The model under review builds one solid part; all positions refer to its coordinate system, in mm. A direction names the side the tool comes from. Give positions to 0.01 mm unless a question says otherwise; leave off trailing zeros. Write each loop counter-clockwise with the first axis right and the second up, starting at its lowest first coordinate (ties: lowest second). Pieces come first, ordered by that corner, then holes. Notation, with made-up numbers: M 25.25,28.25 L 70.25,28.25 A21 ccw 70.25,37.25 Z; hole C -26,41.5 d8. An arc over 180 degrees is marked long. Write item = value, one per line. Start each with the question number.
```python
from build123d import *

# Parameters (mm, degrees)
F0_R        = 1.75
F1_DEPTH    = 1.524
F2_R        = 6.985
F3_T1_DEPTH = 26.7357127365
F4_R        = 4.7625
F5_DEPTH    = 25.4


# Not quite as in the source:
# - a fillet or chamfer that OpenCascade refuses, or shapes differently, is made with other operations: its cross-section is extruded or revolved along the edge and cut away or added


with BuildPart() as f1:
    # F0 (on Top) → F1 (new body)
    with BuildSketch(Plane.XY):
        Polygon((3.175, 3.175), (3.175, 14.2875), (-3.175, 14.2875), (-3.175, 3.175), (-14.2875, 3.175), (-14.2875, -3.175), (-3.175, -3.175), (-3.175, -14.2875), (3.175, -14.2875), (3.175, -3.175), (14.2875, -3.175), (14.2875, 3.175), align=None)
        with BuildLine():
            ThreePointArc((1.75, -9.525), (-1.2374368671, -10.7624368671), (0, -7.775))
            ThreePointArc((0, -7.775), (1.2374368671, -8.2875631329), (1.75, -9.525))
        make_face(mode=Mode.SUBTRACT)
        with Locations((-7.9375, 0)):
            Circle(F0_R, mode=Mode.SUBTRACT)
        with BuildLine():
            ThreePointArc((9.6875, 0), (7.9375, -1.75), (6.1875, 0))
            ThreePointArc((6.1875, 0), (7.9375, 1.75), (9.6875, 0))
        make_face(mode=Mode.SUBTRACT)
        with BuildLine():
            ThreePointArc((0, 7.775), (-1.2374368671, 10.7624368671), (1.75, 9.525))
            ThreePointArc((1.75, 9.525), (1.2374368671, 8.2875631329), (0, 7.775))
        make_face(mode=Mode.SUBTRACT)
    extrude(amount=F1_DEPTH)

    # F2
    f2_edges = [f1.edges().sort_by_distance(p)[0] for p in [
        (3.175, -3.175, 0.762),
        (-3.175, 3.175, 0.762),
        (3.175, 3.175, 0.762),
        (-3.175, -3.175, 0.762),
    ]]
    fillet(f2_edges, radius=F2_R)

    # F3: fillet of radius 5.08 on 8 edges, made by hand

    # F3_s2 → F3_t1 (cut)
    with BuildSketch(Plane.XY.offset(-12.6058563682)):
        with BuildLine():
            ThreePointArc((3.1968016831, 9.6085526316), (1.5800515868, 12.9387027128), (-1.8673425473, 14.2875))
            Line((-1.8673425473, 14.2875), (-1.8673425473, 14.7955))
            Line((-1.8673425473, 14.7955), (3.175, 14.7955))
            Line((3.175, 14.7955), (3.683, 14.2875))
            ThreePointArc((3.683, 14.2875), (3.683, 10.16), (3.7032161062, 9.6486578947))
            Line((3.7032161062, 9.6486578947), (3.1968016831, 9.6085526316))
        make_face()
        with BuildLine():
            ThreePointArc((1.8673425473, 14.2875), (-1.5800515868, 12.9387027128), (-3.1968016831, 9.6085526316))
            Line((-3.1968016831, 9.6085526316), (-3.7032161062, 9.6486578947))
            ThreePointArc((-3.7032161062, 9.6486578947), (-3.683, 10.16), (-3.683, 14.2875))
            Line((-3.683, 14.2875), (-3.175, 14.7955))
            Line((-3.175, 14.7955), (1.8673425473, 14.7955))
            Line((1.8673425473, 14.7955), (1.8673425473, 14.2875))
        make_face()
        with BuildLine():
            ThreePointArc((-14.2875, 1.8673425473), (-12.9387027128, -1.5800515868), (-9.6085526316, -3.1968016831))
            Line((-9.6085526316, -3.1968016831), (-9.6486578947, -3.7032161062))
            ThreePointArc((-9.6486578947, -3.7032161062), (-10.16, -3.683), (-14.2875, -3.683))
            Line((-14.2875, -3.683), (-14.7955, -3.175))
            Line((-14.7955, -3.175), (-14.7955, 1.8673425473))
            Line((-14.7955, 1.8673425473), (-14.2875, 1.8673425473))
        make_face()
        with BuildLine():
            ThreePointArc((-9.6085526316, 3.1968016831), (-12.9387027128, 1.5800515868), (-14.2875, -1.8673425473))
            Line((-14.2875, -1.8673425473), (-14.7955, -1.8673425473))
            Line((-14.7955, -1.8673425473), (-14.7955, 3.175))
            Line((-14.7955, 3.175), (-14.2875, 3.683))
            ThreePointArc((-14.2875, 3.683), (-10.16, 3.683), (-9.6486578947, 3.7032161062))
            Line((-9.6486578947, 3.7032161062), (-9.6085526316, 3.1968016831))
        make_face()
        with BuildLine():
            ThreePointArc((1.8673425473, -14.2875), (-1.5800515868, -12.9387027128), (-3.1968016831, -9.6085526316))
            Line((-3.1968016831, -9.6085526316), (-3.7032161062, -9.6486578947))
            ThreePointArc((-3.7032161062, -9.6486578947), (-3.683, -10.16), (-3.683, -14.2875))
            Line((-3.683, -14.2875), (-3.175, -14.7955))
            Line((-3.175, -14.7955), (1.8673425473, -14.7955))
            Line((1.8673425473, -14.7955), (1.8673425473, -14.2875))
        make_face()
        with BuildLine():
            ThreePointArc((3.1968016831, -9.6085526316), (1.5800515868, -12.9387027128), (-1.8673425473, -14.2875))
            Line((-1.8673425473, -14.2875), (-1.8673425473, -14.7955))
            Line((-1.8673425473, -14.7955), (3.175, -14.7955))
            Line((3.175, -14.7955), (3.683, -14.2875))
            ThreePointArc((3.683, -14.2875), (3.683, -10.16), (3.7032161062, -9.6486578947))
            Line((3.7032161062, -9.6486578947), (3.1968016831, -9.6085526316))
        make_face()
        with BuildLine():
            ThreePointArc((14.2875, 1.8673425473), (12.9387027128, -1.5800515868), (9.6085526316, -3.1968016831))
            Line((9.6085526316, -3.1968016831), (9.6486578947, -3.7032161062))
            ThreePointArc((9.6486578947, -3.7032161062), (10.16, -3.683), (14.2875, -3.683))
            Line((14.2875, -3.683), (14.7955, -3.175))
            Line((14.7955, -3.175), (14.7955, 1.8673425473))
            Line((14.7955, 1.8673425473), (14.2875, 1.8673425473))
        make_face()
        with BuildLine():
            ThreePointArc((9.6085526316, 3.1968016831), (12.9387027128, 1.5800515868), (14.2875, -1.8673425473))
            Line((14.2875, -1.8673425473), (14.7955, -1.8673425473))
            Line((14.7955, -1.8673425473), (14.7955, 3.175))
            Line((14.7955, 3.175), (14.2875, 3.683))
            ThreePointArc((14.2875, 3.683), (10.16, 3.683), (9.6486578947, 3.7032161062))
            Line((9.6486578947, 3.7032161062), (9.6085526316, 3.1968016831))
        make_face()
    extrude(amount=F3_T1_DEPTH, mode=Mode.SUBTRACT)

    # F4 (on face) → F5 (cut)
    with BuildSketch(Plane.XY.offset(1.524)):
        Circle(F4_R)
        with BuildLine():
            ThreePointArc((1.75, 9.525), (0, 11.275), (-1.75, 9.525))
            Line((-1.75, 9.525), (-1.75, 7.775))
            ThreePointArc((-1.75, 7.775), (0, 6.025), (1.75, 7.775))
            Line((1.75, 7.775), (1.75, 9.525))
        make_face()
        with BuildLine():
            ThreePointArc((-1.75, -9.525), (0, -11.275), (1.75, -9.525))
            Line((1.75, -9.525), (1.75, -7.775))
            ThreePointArc((1.75, -7.775), (0, -6.025), (-1.75, -7.775))
            Line((-1.75, -7.775), (-1.75, -9.525))
        make_face()
        with BuildLine():
            ThreePointArc((7.9375, 1.75), (6.1875, 0), (7.9375, -1.75))
            Line((7.9375, -1.75), (9.6875, -1.75))
            ThreePointArc((9.6875, -1.75), (11.4375, 0), (9.6875, 1.75))
            Line((9.6875, 1.75), (7.9375, 1.75))
        make_face()
        with BuildLine():
            ThreePointArc((-7.9375, -1.75), (-6.1875, 0), (-7.9375, 1.75))
            Line((-7.9375, 1.75), (-9.6875, 1.75))
            ThreePointArc((-9.6875, 1.75), (-11.4375, 0), (-9.6875, -1.75))
            Line((-9.6875, -1.75), (-7.9375, -1.75))
        make_face()
    extrude(amount=-F5_DEPTH, mode=Mode.SUBTRACT)


solid = f1.part
```
Item 1: We need section C-C, the plane x = -0.5. Write out the cut boundary in (y, z), and give its area (3 significant figures).
Item 2: We need section B-B, the plane y = -0.5. Write out the cut boundary in (x, z).
Item 3: We need section A-A, the plane z = 0.55. Give the number of separate pieces and of enclosed holes in the cut face, and give its area (3 significant figures).
Item 4: For faces 1 (the flat face through (-1.75, -9, 1)), 2 (the cylindrical face through (-5.27, -5.17, 0.77)), list the 3-axis set-ups (+Z, -Z, +X, -X, +Y, -Y) from which the entire face can be reached by the end or side of a thin tool; tool diameter is ignored.
Item 5: Clearance check with flat-ended pins moving along their axes: P1, Ø0.8, axis at x = 9, z = 0.5, coming from the +Y side; P2, Ø8, axis at x = -7, y = 7, coming from the -Z side; P3, Ø0.8, axis at y = -8.5, z = 0.5, coming from the -X side; P4, Ø5.5, axis at x = 0, y = 0, coming from the +Z side. State where each tip first meets the part, or that it passes through.
Item 6: The part is to be moulded in two halves that separate along Y. For faces 3 (the flat face through (-9, 1.75, 1)), 4 (the cylindrical face through (-0.038, 11.275, 0.751)), 5 (the cylindrical face through (5.27, -5.17, 0.77)), 6 (the cylindrical face through (-2.194, 12.26, 0.751)), say which applies: released by +Y, released by -Y, zero draft, split by the parting line, or undercut.
Item 7: To check wall thickness, follow probe 1 along Y at (x, z) = (0, 0.8) (1 decimal); probe 2 along X at (y, z) = (-1.5, 0.9); probe 3 along X at (y, z) = (0.5, 0.85). State the ranges of each line that lie inside material, in increasing order. Write a range as [from, to].
Worked out:
q1.outline = M -13.7,0 L -11.2,0 L -11.2,1.52 L -13.7,1.52 Z; M -6.1,0 L -4.74,0 L -4.74,1.52 L -6.1,1.52 Z; M 4.74,0 L 6.1,0 L 6.1,1.52 L 4.74,1.52 Z; M 11.2,0 L 13.7,0 L 13.7,1.52 L 11.2,1.52 Z
q1.area = 11.8 mm²
q2.outline = M -13.7,0 L -11.36,0 L -11.36,1.52 L -13.7,1.52 Z; M -6.26,0 L -4.74,0 L -4.74,1.52 L -6.26,1.52 Z; M 4.74,0 L 6.26,0 L 6.26,1.52 L 4.74,1.52 Z; M 11.36,0 L 13.7,0 L 13.7,1.52 L 11.36,1.52 Z
q3.separate_pieces = 1
q3.enclosed_holes = 5
q3.area = 189 mm²
q4.face_1 = +Z, -Z
q4.face_2 = +Z, -Z, -X, -Y
q5.P1 = 3.35
q5.P2 = 0
q5.P3 = -3.49
q5.P4 = through
q6.face_3 = undercut
q6.face_4 = undercut
q6.face_5 = released by -Y
q6.face_6 = released by +Y
q7.probe_1 = [-13.9, -11.3], [-6, -4.8], [4.8, 6], [11.3, 13.9]
q7.probe_2 = [-13.01, -10.59], [-7.04, -4.52], [4.52, 7.04], [10.59, 13.01]
q7.probe_3 = [-13.7, -11.36], [-6.26, -4.74], [4.74, 6.26], [11.36, 13.7]
